```python
from build123d import *

# Parameters (mm, degrees)
EXTRUDE_1_DEPTH = 1.5


with BuildPart() as part:
    # 草图1 → 凸台-拉伸1 (new body)
    with BuildSketch(Plane.XY):
        with BuildLine():
            Line((91.141098719, 85.299098719), (90.976901281, 85.134901281))
            ThreePointArc((90.976901281, 85.134901281), (90.99066635, 85.114300398), (90.9955, 85.09))
            ThreePointArc((90.9955, 85.09), (90.976901281, 85.045098719), (90.932, 85.0265))
            Line((90.932, 85.0265), (90.932, 76.0095))
            ThreePointArc((90.932, 76.0095), (90.976901281, 75.990901281), (90.9955, 75.946))
            Line((90.9955, 75.946), (95.6945, 75.946))
            ThreePointArc((95.6945, 75.946), (95.713098719, 75.990901281), (95.758, 76.0095))
            Line((95.758, 76.0095), (95.758, 82.9945))
            ThreePointArc((95.758, 82.9945), (95.713098719, 83.102901281), (95.8215, 83.058))
            Line((95.8215, 83.058), (97.7265, 83.058))
            ThreePointArc((97.7265, 83.058), (97.79, 83.1215), (97.8535, 83.058))
            Line((97.8535, 83.058), (107.3785, 83.058))
            ThreePointArc((107.3785, 83.058), (107.417699602, 83.11666635), (107.486901281, 83.102901281))
            Line((107.486901281, 83.102901281), (107.651098719, 83.267098719))
            ThreePointArc((107.651098719, 83.267098719), (107.63733365, 83.336300398), (107.696, 83.3755))
            Line((107.696, 83.3755), (107.696, 93.5355))
            ThreePointArc((107.696, 93.5355), (107.63733365, 93.574699602), (107.651098719, 93.643901281))
            Line((107.651098719, 93.643901281), (106.978901281, 94.316098719))
            ThreePointArc((106.978901281, 94.316098719), (106.909699602, 94.30233365), (106.8705, 94.361))
            Line((106.8705, 94.361), (97.7265, 94.361))
            ThreePointArc((97.7265, 94.361), (97.707901281, 94.316098719), (97.663, 94.2975))
            Line((97.663, 94.2975), (97.663, 92.0115))
            ThreePointArc((97.663, 92.0115), (97.707901281, 91.992901281), (97.7265, 91.948))
            ThreePointArc((97.7265, 91.948), (97.707901281, 91.903098719), (97.663, 91.8845))
            Line((97.663, 91.8845), (97.663, 90.4875))
            ThreePointArc((97.663, 90.4875), (97.707901281, 90.468901281), (97.7265, 90.424))
            ThreePointArc((97.7265, 90.424), (97.663, 90.3605), (97.5995, 90.424))
            Line((97.5995, 90.424), (91.2495, 90.424))
            ThreePointArc((91.2495, 90.424), (91.230901281, 90.379098719), (91.186, 90.3605))
            Line((91.186, 90.3605), (91.186, 85.4075))
            ThreePointArc((91.186, 85.4075), (91.230901281, 85.388901281), (91.2495, 85.344))
            ThreePointArc((91.2495, 85.344), (91.210300398, 85.28533365), (91.141098719, 85.299098719))
        make_face()
    extrude(amount=EXTRUDE_1_DEPTH)


solid = part.part
```
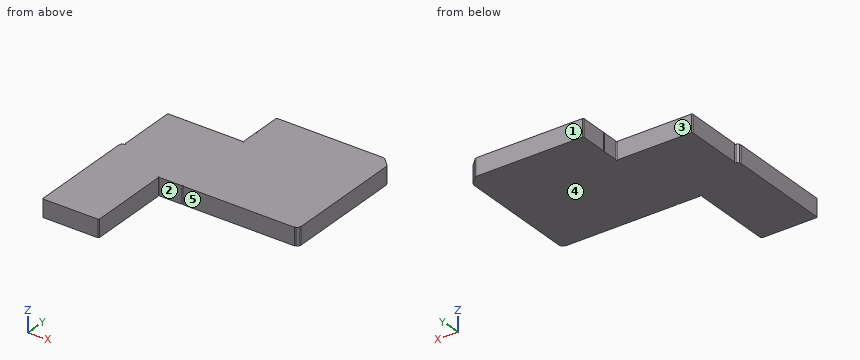
Can you work these out from the model? Positions are in its coordinate system, mm. Face numbers are marked on the shaded views. A direction names the side the tool comes from. Round coordinates to 2 decimals unless told otherwise and drop trailing zeros. Loops run counter-clockwise (first coordinate to the right, second up) from the corner with the lowest first, then second, coordinate; pieces in that order, holes last.
Item 1: Suppose I cut it at C-C, the plane y = 81.5. Write out the boundary of the cut face in (x, z), then the cut area to 3 significant figures.
Item 2: If we mould it in two halves opening along Y, with no side actions, what happens to the marked faces 3, 4 and 5? For each: +Y half, -Y half, draft (parallel to the pull), parting line (faces both ways), or undercut.
Item 3: Suppose I cut it at B-B, the plane x = 96.75. Write out the boundary of the cut face in (y, z), then the cut area to 3 significant figures.
Item 4: Suppose I cut it at A-A, the plane z = 0.4. Write out the boundary of the cut face in (x, y).
Item 5: Please list where these lines run through material, in increasing order: L1, parallel to X at y = 78.25, z = 1; L2, parallel to X at y = 90, z = 0.9; L3, parallel to Y at x = 103.25, z = 1.4.
Item 6: Will this pin go through, and if not, where does the flat tip stop? pin 1 Ø3 at (x, y) = (104, 83) entering from -Z.
Item 7: Which directions (+Z, -Z, +X, -X, +Y, -Y) give clear straight access to the entire face, cutting with the end or side of a thin tool? Please do the marked faces 1 and 2.
Reported:
1. outline: (90.93, 0) - (95.76, 0) - (95.76, 1.5) - (90.93, 1.5) - close
1. area: 7.24 mm2
2. face 3: +Y half
2. face 4: draft
2. face 5: -Y half
3. outline: (83.06, 0) - (90.42, 0) - (90.42, 1.5) - (83.06, 1.5) - close
3. area: 11.0 mm2
4. outline: (90.93, 76.01) arc R0.06 cw to (91, 75.95) - (95.69, 75.95) arc R0.06 cw to (95.76, 76.01) - (95.76, 82.99) arc R0.06 cw (long way) to (95.82, 83.06) - (97.73, 83.06) arc R0.06 cw to (97.85, 83.06) - (107.38, 83.06) arc R0.06 cw to (107.49, 83.1) - (107.65, 83.27) arc R0.06 cw to (107.7, 83.38) - (107.7, 93.54) arc R0.06 cw to (107.65, 93.64) - (106.98, 94.32) arc R0.06 cw to (106.87, 94.36) - (97.73, 94.36) arc R0.06 cw to (97.66, 94.3) - (97.66, 92.01) arc R0.06 cw to (97.66, 91.88) - (97.66, 90.49) arc R0.06 cw (long way) to (97.6, 90.42) - (91.25, 90.42) arc R0.06 cw to (91.19, 90.36) - (91.19, 85.41) arc R0.06 cw (long way) to (91.14, 85.3) - (90.98, 85.13) arc R0.06 cw to (90.93, 85.03) - close
5. L1: x = 90.93 to 95.76
5. L2: x = 91.19 to 107.7
5. L3: y = 83.06 to 94.36
6. pin 1: stops at z = 0
7. face 1: +Z, -Z, +X, -X, +Y
7. face 2: +Z, -Z, +X, -Y
